Source: CAD feature listing. Evaluate the final solid. Frame: model axes, mm. Give positions to 0.01 mm unless a question says otherwise; leave off trailing zeros. Write each loop counter-clockwise with the first axis right and the second up, starting at its lowest first coordinate (ties: lowest second). Pieces come first, ordered by that corner, then holes. Notation, with made-up numbers: (75.5, -25) -> (124.5, -25) arc R29 cw to (124.5, 14) -> close; hole circle Ø7 at (-19, 71.5). An arc over 180 degrees is marked (long way). Use one line per item in the form item = value. Start each with the question number.
(1) Material intervals for line 1 along Z through (x, y) = (63, -40); line 2 along X through (y, z) = (-49, 14); line 3 along Z through (x, y) = (-57, -19), sorted ascending. Write a range as from..to.
(2) Cut plane C-C, the plane y = -29. Output: boundary loops of the cut face in (x, z), and give its area (3 significant figures).
(3) Cut plane A-A, the plane z = 0. Output: boundary loops of the cut face in (x, y), and give its area (3 significant figures).
(4) Cut plane B-B, the plane x = 63.5. Output: boundary loops of the cut face in (y, z).
(5) First-contact query: P1, Ø1, axis at x = -82, z = -60, coming from the +Y side. Flat tip, straight axial feed; report the tip coordinate or a pass-through.
(6) Draft query along Z for faces 1 (the face through (131.54, -25.67, 74.29)), 2 (the face through (15.12, -25.04, -11.59)), 3 (the face through (26, -50.8, 1)). Return one class per face: pulls with the +Z half, pulls with the -Z half, needs draft (parallel to the pull), parting line crosses it, or undercut.
from build123d import *

# Parameters (mm, degrees)
F0_W     = 266.7
F0_H     = 152.4
F1_DEPTH = 50.8
F2_R     = 6.35
F3_R     = 19.05
F4_DEPTH = 63.5


with BuildPart() as f1:
    # F0 (on Front) → F1 (new body)
    with BuildSketch(Plane.XZ):
        Rectangle(F0_W, F0_H)
    extrude(amount=F1_DEPTH)

    # F2
    f2_edges = [f1.edges().sort_by_distance(p)[0] for p in [
        (0, -50.8, 76.2),
        (133.35, -25.4, 76.2),
        (-133.35, -25.4, 76.2),
        (0, 0, 76.2),
        (0, -50.8, -76.2),
        (-133.35, -25.4, -76.2),
        (133.35, -25.4, -76.2),
        (0, 0, -76.2),
        (-133.35, -50.8, 0),
        (-133.35, 0, 0),
        (133.35, -50.8, 0),
        (133.35, 0, 0),
    ]]
    fillet(f2_edges, radius=F2_R)

    # F3 (on face) → F4 (cut)
    with BuildSketch(Plane(origin=(0, 0, 0), x_dir=(-1, 0, 0), z_dir=(0, 1, 0))):
        with Locations((-63.5, 0)):
            Circle(F3_R)
        with BuildLine():
            ThreePointArc((-19.05, 0), (0, -19.05), (19.05, 0))
            Line((19.05, 0), (0, 0))
            Line((0, 0), (-19.05, 0))
        make_face()
        with BuildLine():
            Line((0, 0), (19.05, 0))
            ThreePointArc((19.05, 0), (0, 19.05), (-19.05, 0))
            Line((-19.05, 0), (0, 0))
        make_face()
        with BuildLine():
            ThreePointArc((82.55, 0), (63.5, 19.05), (44.45, 0))
            ThreePointArc((44.45, 0), (63.5, -19.05), (82.55, 0))
        make_face()
    extrude(amount=-F4_DEPTH, mode=Mode.SUBTRACT)


solid = f1.part
Geometry says:
q1.line_1 = -76.2..-19.04, 19.04..76.2
q1.line_2 = -131.43..-76.42, -50.58..-12.92, 12.92..50.58, 76.42..131.43
q1.line_3 = -76.2..-17.91, 17.91..76.2
q2.outline = (-133.35, -69.85) arc R6.35 ccw to (-127, -76.2) -> (127, -76.2) arc R6.35 ccw to (133.35, -69.85) -> (133.35, 69.85) arc R6.35 ccw to (127, 76.2) -> (-127, 76.2) arc R6.35 ccw to (-133.35, 69.85) -> close; hole circle Ø38.1 at (-63.5, 0); hole circle Ø38.1 at (0, 0); hole circle Ø38.1 at (63.5, 0)
q2.area = 37,200 mm^2
q3.outline = (-133.35, -44.45) arc R6.35 ccw to (-127, -50.8) -> (-82.55, -50.8) -> (-82.55, 0) -> (-127, 0) arc R6.35 ccw to (-133.35, -6.35) -> close; (-44.45, -50.8) -> (-19.05, -50.8) -> (-19.05, 0) -> (-44.45, 0) -> close; (19.05, -50.8) -> (44.45, -50.8) -> (44.45, 0) -> (19.05, 0) -> close; (82.55, -50.8) -> (127, -50.8) arc R6.35 ccw to (133.35, -44.45) -> (133.35, -6.35) arc R6.35 ccw to (127, 0) -> (82.55, 0) -> close
q3.area = 7,710 mm^2
q4.outline = (-50.8, -69.85) arc R6.35 ccw to (-44.45, -76.2) -> (-6.35, -76.2) arc R6.35 ccw to (0, -69.85) -> (0, -19.05) -> (-50.8, -19.05) -> close; (-50.8, 19.05) -> (0, 19.05) -> (0, 69.85) arc R6.35 ccw to (-6.35, 76.2) -> (-44.45, 76.2) arc R6.35 ccw to (-50.8, 69.85) -> close
q5.P1 = 0
q6.face_1 = pulls with the +Z half
q6.face_2 = undercut
q6.face_3 = needs draft
